Autodesk Inventor part; units mm, degrees
ref_plane "YZ Plane" through (0, 0, 0) normal (1, 0, 0) x (0, 1, 0)
ref_plane "XZ Plane" through (0, 0, 0) normal (0, 1, 0) x (-1, 0, 0)
ref_plane "XY Plane" through (0, 0, 0) normal (0, 0, 1) x (1, 0, 0)
sketch "Schizzo1" plane through (0, 0, 0) normal (0, 1, 0) x (-1, 0, 0)
  circle A0 centre (0, 0) radius 1
  line L0 (10, 0) -> (10, -10)
  line L1 (10, -10) -> (0, -10)
  line L2 (-10, 0) -> (-10, -10)
  line L3 (-10, -10) -> (0, -10)
  line L4 (10, 0) -> (10, 10)
  line L5 (10, 10) -> (-10, 10)
  line L6 (-10, 10) -> (-10, 0)
  dimension "d2" = 2
  dimension "d12" = 10
  dimension "d13" = 10
  dimension "d14" = 10
  dimension "d15" = 10
extrude "Estrusione2" add sketch "Schizzo1" along normal blind 4
sketch "Schizzo3" plane through (0, 0, 0) normal (0, -1, 0) x (1, 0, 0)
  point P0 (0, 0)
  point P1 (0, 0)
hole "Foro2" at (0, 0, 0) direction (0, 1, 0) diameter 4.5 depth 8 countersink diameter 7 countersink angle 90
properties part number "Fissante"
The model under review builds one solid part; all positions refer to its coordinate system, in mm. Round coordinates to 2 decimals unless told otherwise and drop trailing zeros. Loops run counter-clockwise (first coordinate to the right, second up) from the corner with the lowest first, then second, coordinate; pieces in that order, holes last. Notation, with made-up numbers: (44, -17.75) -> (83, -17.75) arc R33 cw to (83, 13.25) -> close; hole circle Ø2 at (60.5, 84). An arc over 180 degrees is marked (long way). Write item = value, one per line. Start each with the question number.
Item 1: Take a section at B-B on z = 0. Give the boundary of the cut face in (x, y).
Item 2: Take a section at C-C on y = 3.5. Give the boundary of the cut face in (x, z), plus the area to 3 significant figures.
Item 3: Mouldability with a two-part tool opening along Z and no side actions: class faces 1 (the flat face through (10, 2, 0)), 2 (the flat face through (0, 2, 10)), 3 (the cylindrical face through (-2.23, 2.64, 0.29)), 4 (the flat face through (0, 2, -10)) as released by +Z, released by -Z, zero draft, split by the parting line, or undercut.
Item 4: To check wall thickness, follow L1, parallel to Z at x = 0, y = 2.95; L2, parallel to Y at x = 2, z = 2.5. State the ranges of each line that lie inside material, in increasing order.
Item 5: Take a section at A-A on x = 0. Give the boundary of the cut face in (y, z), plus the area to 3 significant figures.
Result:
q1.outline = (-10, 0) -> (-3.5, 0) -> (-2.25, 1.25) -> (-2.25, 4) -> (-10, 4) -> close; (2.25, 1.25) -> (3.5, 0) -> (10, 0) -> (10, 4) -> (2.25, 4) -> close
q2.outline = (-10, -10) -> (10, -10) -> (10, 10) -> (-10, 10) -> close; hole circle Ø4.5 at (0, 0)
q2.area = 384 mm²
q3.face_1 = zero draft
q3.face_2 = released by +Z
q3.face_3 = undercut
q3.face_4 = released by -Z
q4.L1 = -10 to -2.25, 2.25 to 10
q4.L2 = 0.3 to 4
q5.outline = (0, -10) -> (4, -10) -> (4, -2.25) -> (1.25, -2.25) -> (0, -3.5) -> close; (0, 3.5) -> (1.25, 2.25) -> (4, 2.25) -> (4, 10) -> (0, 10) -> close
q5.area = 60.4 mm²
